Verification items for the finished model (mm, model axes). Face numbers are marked on the shaded views. A direction names the side the tool comes from. Give positions to 0.01 mm unless a question says otherwise; leave off trailing zeros. Write each loop counter-clockwise with the first axis right and the second up, starting at its lowest first coordinate (ties: lowest second). Pieces come first, ordered by that corner, then holes.
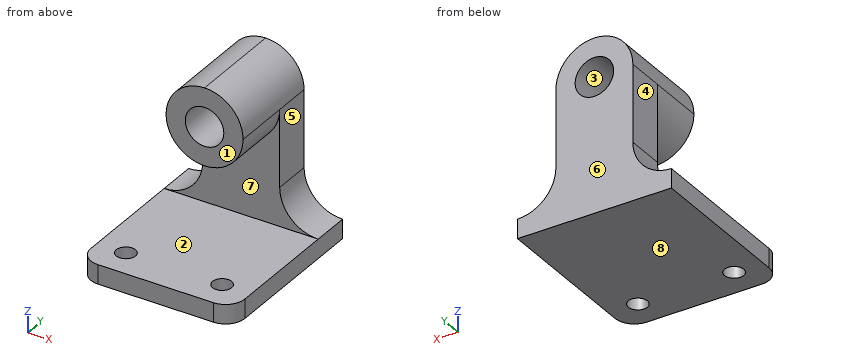
from build123d import *

# Parameters (mm, degrees)
F0_W      = 27.6003498584
F0_H      = 50.8
F0_W_2    = 8.7740728214
F0_W_3    = 14.4255773202
F1_DEPTH  = 31.75
F2_W      = 12.7
F2_H      = 12.7
F3_DEPTH  = 31.751
F4_R      = 6.35
F5_DEPTH  = 31.751
F4_R_2    = 12.7
F6_DEPTH  = 12.7
F8_DEPTH  = 31.751
F10_DEPTH = 19.05
F11_DEPTH = 25.4
F13_DEPTH = 6.351
F14_R     = 3.175
F15_DEPTH = 6.351


with BuildPart() as f1:
    # F0 (on Front) → F1 (new body)
    with BuildSketch(Plane.XZ):
        with Locations((-44.346629642, 31.75)):
            Rectangle(F0_W, F0_H)
        with Locations((-62.5338409818, 31.75)):
            Rectangle(F0_W_2, F0_H)
        with Locations((-23.3336660526, 31.75)):
            Rectangle(F0_W_3, F0_H)
        Polygon((-58.1468045712, 6.35), (-66.9208773925, 6.35), (-66.9208773925, 0), (-16.1208773925, 0), (-16.1208773925, 6.35), (-30.5464547127, 6.35), align=None)
    extrude(amount=F1_DEPTH)

    # F2 (on face) → F3 (cut, through all)
    with BuildSketch(Plane.XZ.offset(31.75)):
        with Locations((-60.5708773925, 50.8)):
            Rectangle(F2_W, F2_H)
        with BuildLine():
            Line((-54.2208773925, 57.15), (-54.2208773925, 44.45))
            ThreePointArc((-54.2208773925, 44.45), (-50.5011335136, 53.4302561211), (-41.5208773925, 57.15))
            Line((-41.5208773925, 57.15), (-54.2208773925, 57.15))
        make_face()
        with BuildLine():
            ThreePointArc((-41.5208773925, 57.15), (-32.5406212715, 53.4302561211), (-28.8208773925, 44.45))
            Line((-28.8208773925, 44.45), (-28.8208773925, 57.15))
            Line((-28.8208773925, 57.15), (-41.5208773925, 57.15))
        make_face()
        with Locations((-22.4708773925, 50.8)):
            Rectangle(F2_W, F2_H)
    extrude(amount=-F3_DEPTH, mode=Mode.SUBTRACT)

    # F4 (on face) → F5 (cut, through all)
    with BuildSketch(Plane.XZ.offset(31.75)):
        with Locations((-41.5208773925, 44.45)):
            Circle(F4_R)
    extrude(amount=-F5_DEPTH, mode=Mode.SUBTRACT)

    # F4 (on face) → F6 (cut)
    with BuildSketch(Plane.XZ.offset(31.75)):
        with Locations((-41.5208773925, 44.45)):
            Circle(F4_R_2)
        with Locations((-41.5208773925, 44.45)):
            Circle(F4_R, mode=Mode.SUBTRACT)
    extrude(amount=F6_DEPTH, mode=Mode.SUBTRACT)

    # F7 (on face) → F8 (cut, through all)
    with BuildSketch(Plane.XZ.offset(31.75)):
        with BuildLine():
            Line((-66.9208773925, 44.45), (-66.9208773925, 6.35))
            ThreePointArc((-66.9208773925, 6.35), (-57.9406212715, 10.0697438789), (-54.2208773925, 19.05))
            Line((-54.2208773925, 19.05), (-54.2208773925, 44.45))
            Line((-54.2208773925, 44.45), (-66.9208773925, 44.45))
        make_face()
        with BuildLine():
            ThreePointArc((-28.8208773925, 19.05), (-25.1011335136, 10.0697438789), (-16.1208773925, 6.35))
            Line((-16.1208773925, 6.35), (-16.1208773925, 44.45))
            Line((-16.1208773925, 44.45), (-28.8208773925, 44.45))
            Line((-28.8208773925, 44.45), (-28.8208773925, 19.05))
        make_face()
    extrude(amount=-F8_DEPTH, mode=Mode.SUBTRACT)

    # F9 (on face) → F10 (cut)
    with BuildSketch(Plane.XZ.offset(31.75)):
        with BuildLine():
            ThreePointArc((-54.2208773925, 19.05), (-57.9406212715, 10.0697438789), (-66.9208773925, 6.35))
            Line((-66.9208773925, 6.35), (-16.1208773925, 6.35))
            ThreePointArc((-16.1208773925, 6.35), (-25.1011335136, 10.0697438789), (-28.8208773925, 19.05))
            Line((-28.8208773925, 19.05), (-28.8208773925, 44.45))
            ThreePointArc((-28.8208773925, 44.45), (-41.5208773925, 31.75), (-54.2208773925, 44.45))
            Line((-54.2208773925, 44.45), (-54.2208773925, 19.05))
        make_face()
    extrude(amount=-F10_DEPTH, mode=Mode.SUBTRACT)

    # F11 (add): a face of the model
    f11_faces = [f1.faces().sort_by_distance(p)[0] for p in [
        (-41.5208773925, -31.75, 3.175),
    ]]
    extrude(f11_faces, amount=F11_DEPTH)

    # F12 (on face) → F13 (cut, through all)
    with BuildSketch(Plane.XY.offset(6.35)):
        with BuildLine():
            Line((-66.9208773925, -50.8), (-66.9208773925, -57.15))
            Line((-66.9208773925, -57.15), (-60.5708773925, -57.15))
            ThreePointArc((-60.5708773925, -57.15), (-65.0610054531, -55.2901280605), (-66.9208773925, -50.8))
        make_face()
        with BuildLine():
            ThreePointArc((-16.1208773925, -50.8), (-17.980749332, -55.2901280605), (-22.4708773925, -57.15))
            Line((-22.4708773925, -57.15), (-16.1208773925, -57.15))
            Line((-16.1208773925, -57.15), (-16.1208773925, -50.8))
        make_face()
    extrude(amount=-F13_DEPTH, mode=Mode.SUBTRACT)

    # F14 (on face) → F15 (cut, through all)
    with BuildSketch(Plane.XY.offset(6.35)):
        with Locations((-57.3958773925, -47.625)):
            Circle(F14_R)
        with Locations((-25.6458773925, -47.625)):
            Circle(F14_R)
    extrude(amount=-F15_DEPTH, mode=Mode.SUBTRACT)


solid = f1.part
Item 1: Sectioned sample at C-C on y = -42. Record the cut outline in (x, z), then the cut area to 3 significant figures.
Answer key:
outline: (-66.92, 0) - (-16.12, 0) - (-16.12, 6.35) - (-66.92, 6.35) - close
area: 323 mm2
Item 2: Release check for a two-part mould opening along Z. For the marked faces 6, 7 and 8 record: released by +Z, released by -Z, zero draft, split by the parting line, or undercut.
Answer key:
face 6: zero draft
face 7: undercut
face 8: released by -Z
Item 3: Scan lines: line 1 along Z through (x, y) = (-46, -45.5); line 2 along Y through (x, z) = (-34.5, 7.5); line 3 along Z through (x, y) = (-43.5, -26). Record each from-to range of solid material in increasing order.
Answer key:
line 1: z = 0 to 6.35
line 2: y = -12.7 to 0
line 3: z = 0 to 6.35, 31.91 to 38.42, 50.48 to 56.99
Item 4: Set-up check for the marked faces 1, 2, 3, 4 and 5: record each of +Z, -Z, +X, -X, +Y, -Y from which the full face is reachable in a straight line by a thin tool's end or side.
Answer key:
face 1: +Z, +X, -X, -Y
face 2: +X, -X, -Y
face 3: +Y, -Y
face 4: +Z, -X, +Y, -Y
face 5: +Z, +X, +Y, -Y
Item 5: Sectioned sample at D-D on z = 34. Record the cut outline in (x, y), then the cut area to 3 significant figures.
Answer key:
outline: (-54.22, -12.7) - (-48.74, -12.7) - (-48.74, -31.75) - (-34.3, -31.75) - (-34.3, -12.7) - (-28.82, -12.7) - (-28.82, 0) - (-54.22, 0) - close
area: 598 mm2
Item 6: Sectioned sample at B-B on x = -28. Record the cut outline in (y, z), then the cut area to 3 significant figures.
Answer key:
outline: (-57.15, 0) - (-49.76, 0) - (-49.76, 6.35) - (-57.15, 6.35) - close; (-45.49, 0) - (0, 0) - (0, 14.56) - (-12.7, 14.56) - (-12.7, 6.35) - (-45.49, 6.35) - close
area: 440 mm2
Item 7: Sectioned sample at A-A on z = 49. Record the cut outline in (x, y), then the cut area to 3 significant figures.
Answer key:
outline: (-53.38, -31.75) - (-45.95, -31.75) - (-45.95, 0) - (-53.38, 0) - close; (-37.09, -31.75) - (-29.66, -31.75) - (-29.66, 0) - (-37.09, 0) - close
area: 472 mm2
Item 8: Depth check by flat-ended pin: pin 1 (11.5 mm diameter, centred on x = -40.5, z = 27, fed in from -Y); pin 2 (4 mm diameter, centred on x = -25.65, y = -47.62, fed in from -Z); pin 3 (10 mm diameter, centred on y = -4, z = 32.5, fed in from +X); pin 4 (1.5 mm diameter, centred on y = -20, z = 37, fed in from +X). Enter the tip coordinate at first touch or a pass-through.
Answer key:
pin 1: stops at y = -31.75
pin 2: passes through
pin 3: stops at x = -28.82
pin 4: stops at x = -30.73
